Geometry check sheet. Reference: the model listing, model coordinates, mm. A direction names the side the tool comes from. Coordinates: 2 decimals unless noted, no trailing zeros. Write each loop counter-clockwise with the first axis right and the second up, starting at its lowest first coordinate (ties: lowest second). Pieces come first, ordered by that corner, then holes. Notation, with made-up numbers: (42, -7) -> (53, -7) arc R11 cw to (53, 1) -> close; hole circle Ø2 at (43, 74.5). An arc over 180 degrees is marked (long way). Use a Markdown table: item, result.
Autodesk Inventor part; units mm, degrees
ref_plane "Work Plane1" through (-153.3, 0, 11) normal (0, 0, 1) x (1, 0, 0)
ref_plane "YZ Plane" through (0, 0, 0) normal (1, 0, 0) x (0, 1, 0)
ref_plane "XZ Plane" through (0, 0, 0) normal (0, 1, 0) x (-1, 0, 0)
sketch "Sketch1" plane through (0, 0, 0) normal (0, 0, 1) x (1, 0, 0)
  line L0 (-153.3, -12.5) -> (-143.3, -12.5)
  line L1 (-143.3, -12.5) -> (-143.3, -11.95)
  line L2 (-143.3, -11.95) -> (-142.1, -11.95)
  line L3 (-142.1, -11.95) -> (-142.1, -12.5)
  line L4 (-142.1, -12.5) -> (-116.3, -12.5)
  line L5 (-116.3, -12.5) -> (-116.3, -13.55)
  line L6 (-116.3, -13.55) -> (127.7, -13.55)
  line L7 (127.7, -13.55) -> (127.7, -12.5)
  line L8 (127.7, -12.5) -> (153.3, -12.5)
  line L9 (153.3, -12.5) -> (153.3, 0)
  line L10 (153.3, 0) -> (-153.3, 0)
  line L11 (-153.3, 0) -> (-153.3, -12.5)
  point P0 (0, 0)
  point P1 (0, 0)
  point P2 (127.7, -13.025)
  point P3 (-153.3, -6.25)
  dimension "d0" = 12.5
  dimension "d1" = 10
  dimension "d2" = 1.2
  dimension "d3" = 0.55
  dimension "d4" = 25.8
  dimension "d5" = 13.55
  dimension "d6" = 11.95
  dimension "d7" = 244
  dimension "d8" = 12.5
  dimension "d26" = 306.6
revolve "Revolution1" add sketch "Sketch1" angle 360 about axis through (153.3, 0, 0) along (-1, 0, 0)
sketch "Sketch2" plane through (-153.3, 0, 0) normal (-1, 0, 0) x (0, 0, 1)
  circle A0 centre (0, 0) radius 11
  point P0 (0, 0)
  dimension "d11" = 22
extrude "Extrusion1" add sketch "Sketch2" along normal blind 64
sketch "Sketch3" plane through (153.3, 0, 0) normal (1, 0, 0) x (0, 0, -1)
  point P0 (0, 0)
sketch "Sketch4" plane through (153.3, 0, 0) normal (1, 0, 0) x (0, 0, -1)
  circle A0 centre (0, 0) radius 11
  point P0 (0, 0)
  dimension "d14" = 22
extrude "Extrusion2" add sketch "Sketch4" along normal blind 69.4
ref_plane "Work Plane1" through (-153.3, 0, 11) normal (0, 0, 1) x (1, 0, 0)
sketch "Sketch5" plane through (-153.3, 0, 11) normal (0, 0, 1) x (1, 0, 0)
  line L0 (-64, 11) -> (-64, -11)
  line L1 (-64, 4) -> (-39, 4)
  line L2 (-39, 4) -> (-39, -4)
  line L3 (-39, -4) -> (-64, -4)
  line L4 (-64, -4) -> (-64, 4)
  circle A0 centre (-39, 0) radius 4
  line L5 (376, -11) -> (376, 11)
  line L6 (376, 4) -> (351, 4)
  line L7 (351, 4) -> (351, -4)
  line L8 (351, -4) -> (376, -4)
  line L9 (376, -4) -> (376, 4)
  circle A1 centre (351, 0) radius 4
  point P0 (153.3, 0)
  point P1 (-64, 0)
  point P2 (376, 0)
  point P3 (376, 0)
  dimension "d17" = 8
  dimension "d18" = 25
  dimension "d19" = 8
  dimension "d20" = 25
extrude "Extrusion3" cut sketch "Sketch5" against normal blind 4
chamfer "Chamfer1" distance 2 angle 45 3 edges at (-217.3, 0, -11) (222.7, -10.8101, -2.0351) (222.7, 10.8101, -2.0351)
chamfer "Chamfer2" distance 5 angle 15 1 edges at (-153.3, 12.5, 0) measured on face at (-149.9667, -12.3381, -2.0051)
chamfer "Chamfer3" distance 5 angle 15 1 edges at (153.3, 12.5, 0) measured on face at (136.2333, -12.3381, -2.0051)
properties part number "Shaft" material "Steel, High Strength, Low Alloy"
Item 1: Section check B-B on x = -176. Record the boundary of the cut face in (y, z), then the cut area to 3 significant figures.
Answer block:
| item | result |
|---|---|
| outline | circle Ø22 at (0, 0) |
| area | 380 mm^2 |
Item 2: Depth check by flat-ended pin: P1, Ø10, axis at x = 160.5, z = 10.5, coming from the -Y side; P2, Ø5, axis at x = -113.5, y = -2.5, coming from the -Z side; P3, Ø1, axis at x = 212.5, z = 8.5, coming from the +Y side; P4, Ø3.5, axis at x = -201, z = 9.5, coming from the +Y side. Enter the tip coordinate at first touch or a pass-through.
Answer block:
| item | result |
|---|---|
| P1 | stops at y = -9.53 |
| P2 | stops at z = -13.55 |
| P3 | stops at y = 7.55 |
| P4 | stops at y = 7.81 |
Item 3: Thickness scan on L1, parallel to Y at x = -84, z = -1.5; L2, parallel to Y at x = -33, z = -6.25; L3, parallel to Z at x = -127.5, y = -1. Record the ranges inside material, lowest first. Write a range as [from, to].
Answer block:
| item | result |
|---|---|
| L1 | y = [-13.47, 13.47] |
| L2 | y = [-12.02, 12.02] |
| L3 | z = [-12.46, 12.46] |
Item 4: Section check A-A on x = -16.5. Record the boundary of the cut face in (y, z), then the cut area to 3 significant figures.
Answer block:
| item | result |
|---|---|
| outline | circle Ø27.1 at (0, 0) |
| area | 577 mm^2 |
Item 5: Tool access check on faces 1 (the cylindrical face through (-142.69, -6.42, -10.08)), 2 (the cylindrical face through (138.144, -11.923, -3.755)), 3 (the cylindrical face through (-145.765, -11.923, -3.755)). Record the directions out of +Z, -Z, +X, -X, +Y, -Y that give a thin tool (end or side, any length) a straight path to the whole face; none if there is none.
Answer block:
| item | result |
|---|---|
| face 1 | none |
| face 2 | +X |
| face 3 | -X |
Item 6: Mould release check, pull along Y, two halves, no side actions. Record for faces 4 (the flat face through (-203, 0, 7)), 5 (the cylindrical face through (7.408, -12.517, 5.19)), 6 (the flat face through (208, 0, 7)), 7 (the flat face through (127.7, -9, -9)): +Y half, -Y half, draft (parallel to the pull), parting line (faces both ways), or undercut.
Answer block:
| item | result |
|---|---|
| face 4 | undercut |
| face 5 | parting line |
| face 6 | undercut |
| face 7 | draft |
